from build123d import *

# Parameters (mm, degrees)
SKETCH_W     = 120
SKETCH_H     = 120
SKETCH_R     = 2.1082
SKETCH_W_2   = 90
SKETCH_H_2   = 90
PAD_DEPTH    = 8.89
SKETCH001_W  = 25.4
SKETCH001_H  = 25.4
SKETCH001_R  = 2.1463
PAD001_DEPTH = 8.89
PAD002_DEPTH = 8.89


with BuildPart() as part:
    # Sketch → Pad (new body)
    with BuildSketch(Plane.XY):
        Rectangle(SKETCH_W, SKETCH_H)
        with Locations((-52.5, 52.5)):
            Circle(SKETCH_R, mode=Mode.SUBTRACT)
        with Locations((52.5, 52.5)):
            Circle(SKETCH_R, mode=Mode.SUBTRACT)
        with Locations((-52.5, -52.5)):
            Circle(SKETCH_R, mode=Mode.SUBTRACT)
        with Locations((52.5, -52.5)):
            Circle(SKETCH_R, mode=Mode.SUBTRACT)
        Rectangle(SKETCH_W_2, SKETCH_H_2, mode=Mode.SUBTRACT)
    extrude(amount=PAD_DEPTH)

    # Sketch001 (on Face13 of Pad) → Pad001 (join)
    with BuildSketch(Plane(origin=(0, 0, 0), x_dir=(1, 0, 0), z_dir=(0, 0, -1))):
        with Locations((-47.3, -72.7)):
            Rectangle(SKETCH001_W, SKETCH001_H)
        with Locations((-47.3, -72.7)):
            Circle(SKETCH001_R, mode=Mode.SUBTRACT)
        with Locations((47.3, -72.7)):
            Rectangle(SKETCH001_W, SKETCH001_H)
        with Locations((47.3, -72.7)):
            Circle(SKETCH001_R, mode=Mode.SUBTRACT)
    extrude(amount=-PAD001_DEPTH)

    # Sketch002 (on Face2 of Pad001) → Pad002 (join)
    with BuildSketch(Plane(origin=(0, 0, 0), x_dir=(1, 0, 0), z_dir=(0, 0, -1))):
        Polygon((-45, 45), (-40.7074, 45), (0, 4.2926), (40.7074, 45), (45, 45), (45, 40.7074), (4.2926, 0), (45, -40.7074), (45, -45), (40.7074, -45), (0, -4.2926), (-40.7074, -45), (-45, -45), (-45, -40.7074), (-4.2926, 0), (-45, 40.7074), align=None)
    extrude(amount=-PAD002_DEPTH)


solid = part.part
Source: CAD feature listing. Evaluate the final solid. Frame: model axes, mm. A direction names the side the tool comes from. Round coordinates to 2 decimals unless told otherwise and drop trailing zeros. Loops run counter-clockwise (first coordinate to the right, second up) from the corner with the lowest first, then second, coordinate; pieces in that order, holes last. Notation, with made-up numbers: (-20, 65.5) - (-14, 65.5) arc R20 cw to (-14, 87.5) - close; hole circle Ø2 at (68.25, -36.75). An arc over 180 degrees is marked (long way). Write item = value, one per line. Start each with the question number.
(1) Section query A-A, the plane y = 66. Output: boundary loops of the cut face in (x, z).
(2) Pull-direction query (Y, two-part tool) for faces 4 (the face through (-47, 85.4, 4)), 5 (the face through (1, -4, 0)), 6 (the face through (-54.173, 51.217, 4.383)); classes: +Y half, -Y half, draft (parallel to the pull), parting line (faces both ways), or undercut.
(3) Set-up query: faces 1 (the face through (0, 60, 4)), 2 (the face through (-20.64, -24.93, 4.38)), 3 (the face through (1, -4, 8.89)). Return all of +Z, -Z, +X, -X, +Y, -Y with unobstructed straight access to the full face (end or side cutting, diameter ignored); none if empty.
(4) Pin query (flat end, axial travel): pin 1 (4.5 mm diameter, centred on x = 17.5, z = 3.5, fed in from +Y); pin 2 (3.5 mm diameter, centred on x = -47.3, y = 72.7, fed in from +Z). Return the tip coordinate at first contact, or that it passes through.
(5) Section query B-B, the plane x = 52.5. Output: boundary loops of the cut face in (y, z).
(6) Section query D-D, the plane y = -52.5. Output: boundary loops of the cut face in (x, z).
(7) Section query C-C, the plane z = 6. State how many separate pieces and enclosed holes the cut face has, plus the area to 3 significant figures.
(8) Ray query, line 1 along X through (y, z) = (72.7, 4.5); line 2 along Y through (x, z) = (52.5, 2); line 3 along Y through (x, z) = (47.3, 4). Return the intervals inside material, ascending. Write a range as from..to.
Conclusion:
q1.outline = (-60, 0) - (-34.6, 0) - (-34.6, 8.89) - (-60, 8.89) - close; (34.6, 0) - (60, 0) - (60, 8.89) - (34.6, 8.89) - close
q2.face_4 = +Y half
q2.face_5 = draft
q2.face_6 = undercut
q3.face_1 = +Z, -Z, +Y
q3.face_2 = +Z, -Z
q3.face_3 = +Z, +X, -X, +Y, -Y
q4.pin_1 = 60
q4.pin_2 = through
q5.outline = (-60, 0) - (-54.61, 0) - (-54.61, 8.89) - (-60, 8.89) - close; (-50.39, 0) - (50.39, 0) - (50.39, 8.89) - (-50.39, 8.89) - close; (54.61, 0) - (85.4, 0) - (85.4, 8.89) - (54.61, 8.89) - close
q6.outline = (-60, 0) - (-54.61, 0) - (-54.61, 8.89) - (-60, 8.89) - close; (-50.39, 0) - (50.39, 0) - (50.39, 8.89) - (-50.39, 8.89) - close; (54.61, 0) - (60, 0) - (60, 8.89) - (54.61, 8.89) - close
q7.separate_pieces = 1
q7.enclosed_holes = 10
q7.area = 8,980 mm2
q8.line_1 = -60..-49.45, -45.15..-34.6, 34.6..45.15, 49.45..60
q8.line_2 = -60..-54.61, -50.39..50.39, 54.61..85.4
q8.line_3 = -60..70.55, 74.85..85.4
